from build123d import *

# Parameters (mm, degrees)
SKETCH1_W           = 184.061364714
SKETCH1_H           = 55.833983991
SKETCH1_R           = 8
SKETCH1_R_2         = 2.5
SKETCH1_R_3         = 2
SKETCH1_R_4         = 7
SKETCH1_W_2         = 4
SKETCH1_H_2         = 6
SKETCH1_W_3         = 3
SKETCH1_H_3         = 7
BOSS_EXTRUDE1_DEPTH = 4


with BuildPart() as part:
    # Sketch1 → Boss-Extrude1 (new body)
    with BuildSketch(Plane(origin=(0, 0, 0), x_dir=(1, 0, 0), z_dir=(0, 1, 0))):
        with Locations((0, 7.472529138)):
            Rectangle(SKETCH1_W, SKETCH1_H)
        with Locations(Location((0, 24, 0), (0, 0, 270))):
            Circle(SKETCH1_R, mode=Mode.SUBTRACT)
        with Locations(Location((0, 0, 0), (0, 0, 270))):
            Circle(SKETCH1_R, mode=Mode.SUBTRACT)
        with Locations(Location((-57.4, -5.031515304, 0), (0, 0, 270))):
            Circle(SKETCH1_R_2, mode=Mode.SUBTRACT)
        with Locations(Location((-47.507878323, -13.796629956, 0), (0, 0, 270))):
            Circle(SKETCH1_R_3, mode=Mode.SUBTRACT)
        with Locations(Location((-47.507878323, 4.203370044, 0), (0, 0, 270))):
            Circle(SKETCH1_R_3, mode=Mode.SUBTRACT)
        with Locations(Location((-59.862251394, 13.632128132, 0), (0, 0, 270))):
            Circle(SKETCH1_R_3, mode=Mode.SUBTRACT)
        with Locations(Location((-64.841917038, 30.968484696, 0), (0, 0, 270))):
            Circle(SKETCH1_R_3, mode=Mode.SUBTRACT)
        with Locations(Location((-72.341917038, 30.968484696, 0), (0, 0, 270))):
            Circle(SKETCH1_R_3, mode=Mode.SUBTRACT)
        with Locations(Location((-79.841917038, 30.968484696, 0), (0, 0, 270))):
            Circle(SKETCH1_R_3, mode=Mode.SUBTRACT)
        with Locations(Location((-68, -5.031515304, 0), (0, 0, 270))):
            Circle(SKETCH1_R_4, mode=Mode.SUBTRACT)
        with Locations(Location((-51.349592133, 15.545742715, 0), (0, 0, 270))):
            Circle(SKETCH1_R_3, mode=Mode.SUBTRACT)
        with Locations(Location((51.349592133, 15.545742715, 0), (0, 0, 90))):
            Circle(SKETCH1_R_3, mode=Mode.SUBTRACT)
        with Locations(Location((68, -5.031515304, 0), (0, 0, 90))):
            Circle(SKETCH1_R_4, mode=Mode.SUBTRACT)
        with Locations(Location((79.841917038, 30.968484696, 0), (0, 0, 90))):
            Circle(SKETCH1_R_3, mode=Mode.SUBTRACT)
        with Locations(Location((72.341917038, 30.968484696, 0), (0, 0, 90))):
            Circle(SKETCH1_R_3, mode=Mode.SUBTRACT)
        with Locations(Location((64.841917038, 30.968484696, 0), (0, 0, 90))):
            Circle(SKETCH1_R_3, mode=Mode.SUBTRACT)
        with Locations(Location((59.862251394, 13.632128132, 0), (0, 0, 90))):
            Circle(SKETCH1_R_3, mode=Mode.SUBTRACT)
        with Locations(Location((47.507878323, 4.203370044, 0), (0, 0, 90))):
            Circle(SKETCH1_R_3, mode=Mode.SUBTRACT)
        with Locations(Location((47.507878323, -13.796629956, 0), (0, 0, 90))):
            Circle(SKETCH1_R_3, mode=Mode.SUBTRACT)
        with Locations(Location((57.4, -5.031515304, 0), (0, 0, 90))):
            Circle(SKETCH1_R_2, mode=Mode.SUBTRACT)
        with BuildLine():
            Line((-5, 15.5), (-5, 8.5))
            ThreePointArc((-5, 8.5), (-7.5, 6), (-10, 8.5))
            Line((-10, 8.5), (-10, 15.5))
            ThreePointArc((-10, 15.5), (-7.5, 18), (-5, 15.5))
        make_face(mode=Mode.SUBTRACT)
        with Locations((-33, -5.031515304)):
            Rectangle(SKETCH1_W_2, SKETCH1_H_2, mode=Mode.SUBTRACT)
        with BuildLine():
            Line((5, 15.5), (5, 8.5))
            ThreePointArc((5, 8.5), (7.5, 6), (10, 8.5))
            Line((10, 8.5), (10, 15.5))
            ThreePointArc((10, 15.5), (7.5, 18), (5, 15.5))
        make_face(mode=Mode.SUBTRACT)
        with Locations((33, -5.031515304)):
            Rectangle(SKETCH1_W_2, SKETCH1_H_2, mode=Mode.SUBTRACT)
        with Locations((78.341917038, 10.468484696)):
            Rectangle(SKETCH1_W_3, SKETCH1_H_3, mode=Mode.SUBTRACT)
        Polygon((-72.090338009, 18.166660574), (-74.018700838, 20.464793903), (-81.679145269, 14.036917806), (-79.75078244, 11.738784477), align=None, mode=Mode.SUBTRACT)
        with BuildLine():
            Line((-88.619268655, 19.962128437), (-84.023001996, 23.818854095))
            ThreePointArc((-84.023001996, 23.818854095), (-81.20533789, 23.572340428), (-81.451851557, 20.754676323))
            Line((-81.451851557, 20.754676323), (-86.048118216, 16.897950664))
            ThreePointArc((-86.048118216, 16.897950664), (-88.865782322, 17.144464331), (-88.619268655, 19.962128437))
        make_face(mode=Mode.SUBTRACT)
    extrude(amount=BOSS_EXTRUDE1_DEPTH)


solid = part.part
The listing builds one solid part. Answer for the finished solid, in the listing's coordinates (mm). Give positions to 0.01 mm unless a question says otherwise; leave off trailing zeros. Write each loop counter-clockwise with the first axis right and the second up, starting at its lowest first coordinate (ties: lowest second). Pieces come first, ordered by that corner, then holes.
1) Section A-A (x = 0) is taken. Write down the section's boundary in (y, z), and give its area (3 significant figures).
2) For a pull along X with two mould halves and no side action, classify faces 1 (the face through (-1, 4, -14)), 2 (the face through (-92.031, 2, -7)), 3 (the face through (78, 2, -6.968)) as pulls with the +X half, pulls with the -X half, needs draft (parallel to the pull), parting line crosses it, or undercut.
3) Given P1, Ø2.5, axis at x = -47.51, z = -4.2, coming from the +Y side, flat-ended and moving along its own axis, determine where the tip first touches the part or whether it passes through.
4) Section B-B (z = 5) is taken. Count the separate pieces of the cut face and the enclosed holes in it, and give its area (3 significant figures).
5) Find the intervals of material crossed by L1, parallel to X at y = 0.2, z = 13.5; L2, parallel to X at y = 0.3, z = 13; L3, parallel to X at y = 1.95, z = -0.5, in increasing order.
Response:
1. outline: (0, -35.39) - (4, -35.39) - (4, -32) - (0, -32) - close; (0, -16) - (4, -16) - (4, -8) - (0, -8) - close; (0, 8) - (4, 8) - (4, 20.44) - (0, 20.44) - close
1. area: 95.3 mm2
2. face 1: needs draft
2. face 2: pulls with the -X half
2. face 3: undercut
3. P1: passes through
4. separate pieces: 8
4. enclosed holes: 0
4. area: 502 mm2
5. L1: x = -92.03 to -49.49, -45.53 to 45.53, 49.49 to 92.03
5. L2: x = -92.03 to -49.34, -45.67 to 45.67, 49.34 to 92.03
5. L3: x = -92.03 to -72.29, -63.71 to -7.98, 7.98 to 63.71, 72.29 to 92.03
